Geometry: see drawing. Coordinates: mm, zero at the bounding-box minimum. A direction names the side the tool comes from. Coordinates: 2 decimals unless noted, no trailing zeros. Loops run counter-clockwise (first coordinate to the right, second up) from the corner with the lowest first, then second, coordinate; pieces in that order, holes last.
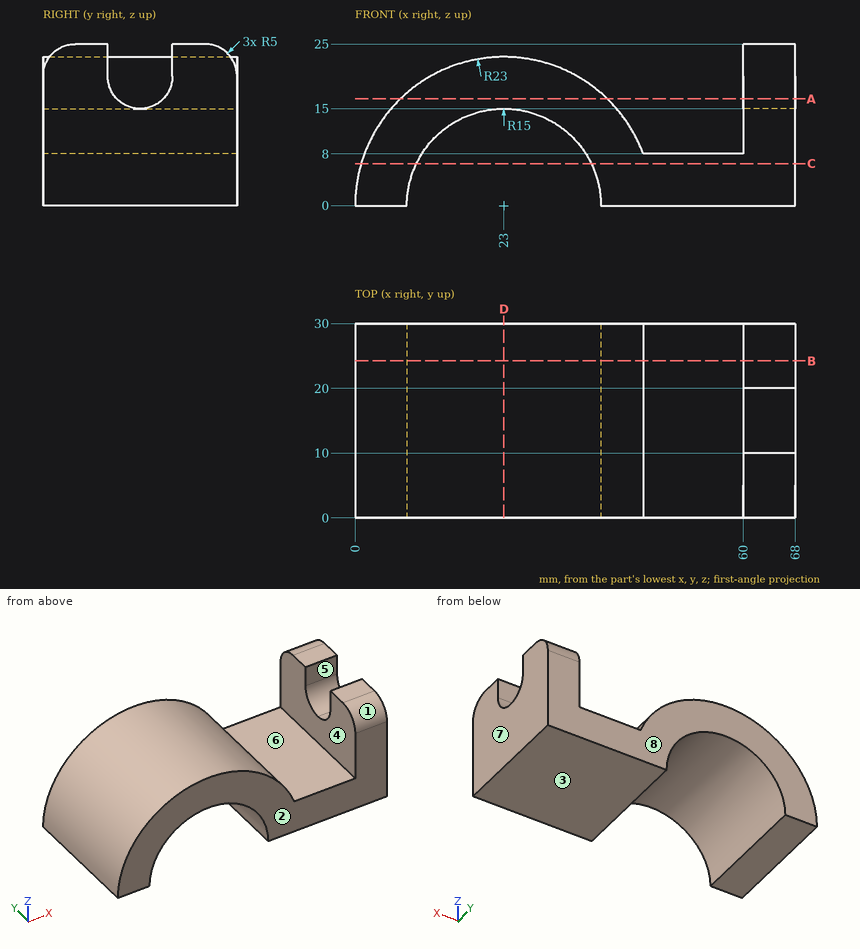
Item 1: Section query A-A (z = 16.5). Output: boundary loops of the cut face in (x, y).
Result:
outline: (6.98, 0) - (39.02, 0) - (39.02, 30) - (6.98, 30) - close; (60, 0) - (68, 0) - (68, 11.43) - (60, 11.43) - close; (60, 18.57) - (68, 18.57) - (68, 30) - (60, 30) - close
Item 2: Section query D-D (x = 23). Output: boundary loops of the cut face in (y, z).
Result:
outline: (0, 15) - (30, 15) - (30, 23) - (0, 23) - close
Item 3: Reachability of the marked faces 1, 2, 3, 4 and 5 from +Z, -Z, +X, -X, +Y, -Y: full face, straight path, thin tool, end or side. Return the list, or none.
Result:
face 1: +Z, +X, -Y
face 2: +Z, -Z, +X, -X, -Y
face 3: -Z, +X, -X, +Y, -Y
face 4: +Z, +Y, -Y
face 5: +Z, +X
Item 4: Section query C-C (z = 6.5). Output: boundary loops of the cut face in (x, y).
Result:
outline: (0.94, 0) - (9.48, 0) - (9.48, 30) - (0.94, 30) - close; (36.52, 0) - (68, 0) - (68, 30) - (36.52, 30) - close
Item 5: Mould query, pull axis X, two halves, no side actions, for the marked faces 6, 7 and 8. Classes: +X half, -X half, draft (parallel to the pull), parting line (faces both ways), or undercut.
Result:
face 6: undercut
face 7: +X half
face 8: draft
Item 6: Line query: L1, parallel to X at y = 22, z = 10.25; L2, parallel to X at y = 18.75, z = 8.5; L3, parallel to Z at x = 49, y = 12.5. Output: solid intervals per line, ascending.
Result:
L1: x = 2.41 to 12.05, 33.95 to 43.59, 60 to 68
L2: x = 1.63 to 10.64, 35.36 to 44.37, 60 to 68
L3: z = 0 to 8
Item 7: Contact query for flat-ended pins moving along their axis: P1, Ø4, axis at x = 65.5, z = 23.5, coming from the -Y side; P2, Ø5.5, axis at x = 65.5, z = 23.5, coming from the +Y side; P3, Ø2, axis at x = 28.5, y = 7, coming from the -Z side; P4, Ø17, axis at x = 53.5, y = 19, coming from the +Z side. Output: stop coordinate, or through.
Result:
P1: stops at y = 0.23
P2: stops at y = 29.94
P3: stops at z = 13.52
P4: stops at z = 25
Item 8: Section query B-B (y = 24.25). Output: boundary loops of the cut face in (x, z).
Result:
outline: (0, 0) - (8, 0) arc R15 cw to (38, 0) - (68, 0) - (68, 25) - (60, 25) - (60, 8) - (44.56, 8) arc R23 ccw to start
